from build123d import *

# Parameters (mm, degrees)
SKETCH1_W           = 20
SKETCH1_H           = 20
BOSS_EXTRUDE1_DEPTH = 10
SKETCH3_W           = 10
SKETCH3_H           = 10
CUT_EXTRUDE1_DEPTH  = 111
SKETCH4_W           = 35
SKETCH4_H           = 3
BOSS_EXTRUDE2_DEPTH = 10


with BuildPart() as part:
    # Sketch1 → Boss-Extrude1 (new body, symmetric)
    with BuildSketch(Plane(origin=(0, 0, 0), x_dir=(1, 0, 0), z_dir=(0, 1, 0))):
        Polygon((10, 35), (10, -35), (10, -55), (18, -55), (18, 55), (10, 55), align=None)
        with Locations((0, -45)):
            Rectangle(SKETCH1_W, SKETCH1_H)
        with Locations((0, 45)):
            Rectangle(SKETCH1_W, SKETCH1_H)
    extrude(amount=BOSS_EXTRUDE1_DEPTH, both=True)

    # Sketch3 → Cut-Extrude1 (cut, through all)
    with BuildSketch(Plane.XY.offset(55)):
        Rectangle(SKETCH3_W, SKETCH3_H)
    extrude(amount=-CUT_EXTRUDE1_DEPTH, mode=Mode.SUBTRACT)

    # Sketch4 → Boss-Extrude2 (add, symmetric)
    with BuildSketch(Plane(origin=(0, 0, 0), x_dir=(1, 0, 0), z_dir=(0, 1, 0))):
        Polygon((-10, -38), (-10, -35), (-18, -35), (-18, -38), (-23, -38), (-23, -35), (-45, -35), (-45, -38), (-28, -38), (-28, -41), (-13, -41), (-13, -38), align=None)
        with Locations((-27.5, 36.5)):
            Rectangle(SKETCH4_W, SKETCH4_H)
    extrude(amount=BOSS_EXTRUDE2_DEPTH, both=True)


solid = part.part
Part model, mm, in its own coordinate system. A direction names the side the tool comes from. Give positions to 0.01 mm unless a question says otherwise; leave off trailing zeros. Order: outer loops, then holes, each group sorted by start corner. A loop starts at its lowest first (then second) coordinate and runs counter-clockwise, first axis right, second up. Notation, with made-up numbers: (88, -38.75) -> (137, -38.75) arc R32 ccw to (137, -9.75) -> close; hole circle Ø10 at (46, -37.5). An arc over 180 degrees is marked (long way). Use one line per item in the form item = value.
(1) Flat gauge pins, fed straight in: P1, Ø5.5, axis at x = -19.5, y = -1, coming from the -Z side; P2, Ø3, axis at y = 1.5, z = 25, coming from the -X side; P3, Ø7.5, axis at x = -23.5, y = -1, coming from the +Z side; P4, Ø10, axis at x = -11, z = 42.5, coming from the +Y side. Where does each tip first touch, or does it go through?
Solution:
P1 = -38
P2 = 10
P3 = 41
P4 = 10
(2) Saw through at A-A (x = -34). Write the cut outline in (y, z), then the cut area to 3 significant figures.
Solution:
outline = (-10, -38) -> (10, -38) -> (10, -35) -> (-10, -35) -> close; (-10, 35) -> (10, 35) -> (10, 38) -> (-10, 38) -> close
area = 120 mm²
(3) Drill centre lines: line 1 (X direction, y = -2.5, z = 36); line 2 (Z direction, x = -12, y = 1.5); line 3 (Z direction, x = -27, y = -1). Where is each one in solid material? Low to high. Write a range as from..to.
Solution:
line_1 = -45..-23, -18..-5, 5..18
line_2 = -38..-35, 35..38
line_3 = -38..-35, 35..41
(4) Saw through at B-B (y = 0.25). Write the cut outline in (x, z).
Solution:
outline = (-45, -38) -> (-10, -38) -> (-10, -55) -> (-5, -55) -> (-5, -35) -> (-45, -35) -> close; (-45, 35) -> (-23, 35) -> (-23, 38) -> (-18, 38) -> (-18, 35) -> (-5, 35) -> (-5, 55) -> (-10, 55) -> (-10, 38) -> (-13, 38) -> (-13, 41) -> (-28, 41) -> (-28, 38) -> (-45, 38) -> close; (5, -55) -> (18, -55) -> (18, 55) -> (5, 55) -> (5, 35) -> (10, 35) -> (10, -35) -> (5, -35) -> close
(5) Pull direction Y, two halves, no side cores. Call faces 1 (the face through (14, 10, -1)), 2 (the face through (18, 0, 1)), 3 (the face through (0, 5, -45)): +Y half, -Y half, draft (parallel to the pull), parting line (faces both ways), or undercut.
Solution:
face_1 = +Y half
face_2 = draft
face_3 = undercut
(6) Saw through at D-D (y = 7.25). Write the cut outline in (x, z), then the cut area to 3 significant figures.
Solution:
outline = (-45, -38) -> (-10, -38) -> (-10, -55) -> (18, -55) -> (18, 55) -> (-10, 55) -> (-10, 38) -> (-13, 38) -> (-13, 41) -> (-28, 41) -> (-28, 38) -> (-45, 38) -> (-45, 35) -> (-23, 35) -> (-23, 38) -> (-18, 38) -> (-18, 35) -> (10, 35) -> (10, -35) -> (-45, -35) -> close
area = 1,920 mm²
(7) Tool access for faces 4 (the face through (-23, 0, 37)), 5 (the face through (-37, 0, 38)), 6 (the face through (-18, 0, -35)), 7 (the face through (-5, 0, 45)): list every direction of +Z, -Z, +X, -X, +Y, -Y with a clear straight run to the whole face (end or side of a thin tool).
Solution:
face_4 = +Y, -Y
face_5 = +Z, -X, +Y, -Y
face_6 = -X, +Y, -Y
face_7 = +Z, -Z
(8) Saw through at C-C (x = 1). Write the cut outline in (y, z), then the cut area to 3 significant figures.
Solution:
outline = (-10, -55) -> (-5, -55) -> (-5, -35) -> (-10, -35) -> close; (-10, 35) -> (-5, 35) -> (-5, 55) -> (-10, 55) -> close; (5, -55) -> (10, -55) -> (10, -35) -> (5, -35) -> close; (5, 35) -> (10, 35) -> (10, 55) -> (5, 55) -> close
area = 400 mm²
